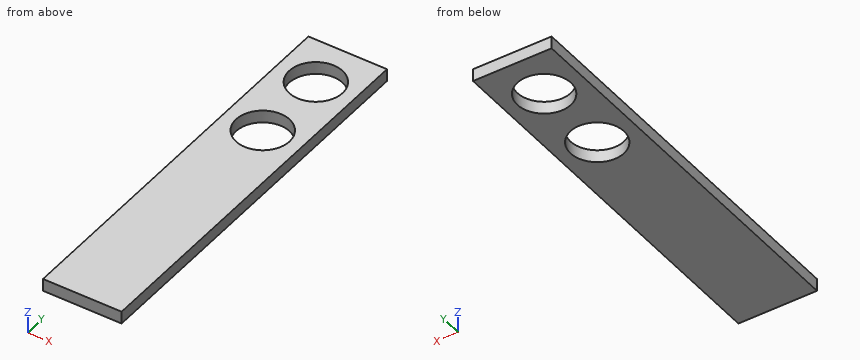
```python
from build123d import *

# Parameters (mm, degrees)
SKETCH1_W            = 5
SKETCH1_H            = 25
BOSS_EXTRUDE1_DEPTH  = 0.79375
M3_CLEARANCE_HOLE1_D = 3.4


with BuildPart() as part:
    # Sketch1 → Boss-Extrude1 (new body)
    with BuildSketch(Plane.XY):
        with Locations((0.590659341, -7.953296703)):
            Rectangle(SKETCH1_W, SKETCH1_H)
    extrude(amount=BOSS_EXTRUDE1_DEPTH)

    # M3 Clearance Hole1 (through all)
    with Locations(Plane(origin=(0, 0, 0), x_dir=(-1, 0, 0), z_dir=(0, 0, -1))):
        with Locations((-0.590659341, 1.546703297), (-0.590659341, -3.453296703)):
            Hole(M3_CLEARANCE_HOLE1_D / 2)


solid = part.part
```
The listing builds one solid part. Answer for the finished solid, in the listing's coordinates (mm). Give positions to 0.01 mm unless a question says otherwise; leave off trailing zeros. Write each loop counter-clockwise with the first axis right and the second up, starting at its lowest first coordinate (ties: lowest second). Pieces come first, ordered by that corner, then holes. Notation, with made-up numbers: (-28.75, 82.5) - (28.25, 82.5) arc R14 ccw to (28.25, 99.5) - close; hole circle Ø1 at (39, 75). An arc over 180 degrees is marked (long way). Use one line per item in the form item = value. Start each with the question number.
1) Consider line 1 along Y through (x, z) = (-0.7, 0.75); line 2 along Y through (x, z) = (1.1, 0.5); line 3 along X through (y, z) = (3, 0.75). Determine where each line is inside the solid, lowest interval first. Write a range as from..to.
2) Find section A-A on x = 0.2. Determine the outline of the cut face in (y, z).
3) Find section B-B on y = -2.75. Determine the outline of the cut face in (x, z), plus the area to 3 significant figures.
4) Find section C-C on x = -0.9. Determine the outline of the cut face in (y, z).
Geometry results:
q1.line_1 = -20.45..-4.56, -2.35..0.44, 2.65..4.55
q1.line_2 = -20.45..-5.08, -1.83..-0.08, 3.17..4.55
q1.line_3 = -1.91..-0.29, 1.47..3.09
q2.outline = (-20.45, 0) - (-5.11, 0) - (-5.11, 0.79) - (-20.45, 0.79) - close; (-1.8, 0) - (-0.11, 0) - (-0.11, 0.79) - (-1.8, 0.79) - close; (3.2, 0) - (4.55, 0) - (4.55, 0.79) - (3.2, 0.79) - close
q3.outline = (-1.91, 0) - (-0.96, 0) - (-0.96, 0.79) - (-1.91, 0.79) - close; (2.14, 0) - (3.09, 0) - (3.09, 0.79) - (2.14, 0.79) - close
q3.area = 1.51 mm2
q4.outline = (-20.45, 0) - (-4.27, 0) - (-4.27, 0.79) - (-20.45, 0.79) - close; (-2.64, 0) - (0.73, 0) - (0.73, 0.79) - (-2.64, 0.79) - close; (2.36, 0) - (4.55, 0) - (4.55, 0.79) - (2.36, 0.79) - close
